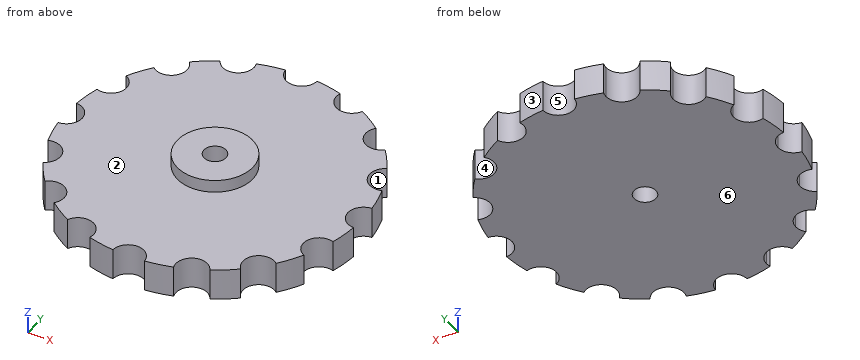
```python
from build123d import *

# Parameters (mm, degrees)
F1_DEPTH = 5
F2_R     = 6
F3_DEPTH = 2
F4_R     = 1.75
F5_DEPTH = 25


with BuildPart() as f1:
    # F0 (on Top) → F1 (new body)
    with BuildSketch(Plane.XY):
        with BuildLine():
            ThreePointArc((23.3670212736, -2.4964608548), (21, -2.53e-08), (23.3670212796, 2.4964607985))
            ThreePointArc((23.3670212796, 2.4964607985), (23.0484540943, 4.5846225431), (22.5436668971, 6.6357428244))
            ThreePointArc((22.5436668971, 6.6357428244), (19.40147019, 8.0363520621), (20.6329585055, 11.2486009491))
            ThreePointArc((20.6329585055, 11.2486009491), (19.5395358989, 13.0559004612), (18.2882435892, 14.7577148103))
            ThreePointArc((18.2882435892, 14.7577148103), (14.8492424139, 14.849242396), (14.7577148323, 18.2882435714))
            ThreePointArc((14.7577148323, 18.2882435714), (13.0559004848, 19.5395358832), (11.248600974, 20.6329584919))
            ThreePointArc((11.248600974, 20.6329584919), (8.0363520855, 19.4014701803), (6.6357428516, 22.5436668891))
            ThreePointArc((6.6357428516, 22.5436668891), (4.5846225709, 23.0484540888), (2.4964608267, 23.3670212766))
            ThreePointArc((2.4964608267, 23.3670212766), (0, 21), (-2.4964608267, 23.3670212766))
            ThreePointArc((-2.4964608267, 23.3670212766), (-4.5846225153, 23.0484540998), (-6.6357427429, 22.5436669211))
            ThreePointArc((-6.6357427429, 22.5436669211), (-6.5289892822, 22.1334873299), (-6.4930605625, 21.7111690547))
            ThreePointArc((-6.4930605625, 21.7111690547), (-8.440272529, 19.2730498225), (-11.2486008745, 20.6329585461))
            ThreePointArc((-11.2486008745, 20.6329585461), (-13.0559003906, 19.5395359461), (-14.7577147442, 18.2882436426))
            ThreePointArc((-14.7577147442, 18.2882436426), (-14.2826746546, 17.5119294358), (-14.1170092878, 16.617009428))
            ThreePointArc((-14.1170092878, 16.617009428), (-15.5991894549, 14.3335815688), (-18.2882435181, 14.7577148984))
            ThreePointArc((-18.2882435181, 14.7577148984), (-19.539535836, 13.0559005554), (-20.6329584512, 11.2486010486))
            ThreePointArc((-20.6329584512, 11.2486010486), (-19.5962781638, 10.3261912121), (-19.2111689788, 8.9930607456))
            ThreePointArc((-19.2111689788, 8.9930607456), (-20.267431592, 6.9520751117), (-22.5436668651, 6.6357429331))
            ThreePointArc((-22.5436668651, 6.6357429331), (-23.0484540722, 4.5846226542), (-23.3670212676, 2.4964609112))
            ThreePointArc((-23.3670212676, 2.4964609112), (-21.6858270712, 1.7201095537), (-21, 8.5e-08))
            ThreePointArc((-21, 8.5e-08), (-21.6858270774, -1.7201093903), (-23.3670212856, -2.4964607422))
            ThreePointArc((-23.3670212856, -2.4964607422), (-23.0484541054, -4.5846224875), (-22.5436669131, -6.6357427701))
            ThreePointArc((-22.5436669131, -6.6357427701), (-20.2674316496, -6.9520749599), (-19.2111690438, -8.9930605886))
            ThreePointArc((-19.2111690438, -8.9930605886), (-19.5962782336, -10.3261910627), (-20.6329585326, -11.2486008994))
            ThreePointArc((-20.6329585326, -11.2486008994), (-19.5395359304, -13.0559004141), (-18.2882436248, -14.7577147662))
            ThreePointArc((-18.2882436248, -14.7577147662), (-15.5991895668, -14.3335814524), (-14.1170094079, -16.6170093078))
            ThreePointArc((-14.1170094079, -16.6170093078), (-14.282674778, -17.5119293241), (-14.7577148764, -18.2882435359))
            ThreePointArc((-14.7577148764, -18.2882435359), (-13.0559005319, -19.5395358517), (-11.2486010237, -20.6329584648))
            ThreePointArc((-11.2486010237, -20.6329584648), (-8.4402726772, -19.2730497595), (-6.4930607194, -21.7111689896))
            ThreePointArc((-6.4930607194, -21.7111689896), (-6.5289894407, -22.1334872737), (-6.6357429059, -22.5436668731))
            ThreePointArc((-6.6357429059, -22.5436668731), (-4.5846226264, -23.0484540777), (-2.496460883, -23.3670212706))
            ThreePointArc((-2.496460883, -23.3670212706), (-5.06e-08, -21), (2.4964607704, -23.3670212826))
            ThreePointArc((2.4964607704, -23.3670212826), (4.5846225153, -23.0484540998), (6.6357427973, -22.5436669051))
            ThreePointArc((6.6357427973, -22.5436669051), (8.0363520388, -19.4014701997), (11.2486009242, -20.632958519))
            ThreePointArc((11.2486009242, -20.632958519), (13.0559004377, -19.5395359147), (14.7577147882, -18.288243607))
            ThreePointArc((14.7577147882, -18.288243607), (14.8492423781, -14.8492424318), (18.2882435536, -14.7577148544))
            ThreePointArc((18.2882435536, -14.7577148544), (19.5395358675, -13.0559005083), (20.6329584783, -11.2486009988))
            ThreePointArc((20.6329584783, -11.2486009988), (19.4014701706, -8.0363521089), (22.5436668811, -6.6357428788))
            ThreePointArc((22.5436668811, -6.6357428788), (23.0484540833, -4.5846225986), (23.3670212736, -2.4964608548))
        make_face()
    extrude(amount=F1_DEPTH)

    # F2 (on face) → F3 (join)
    with BuildSketch(Plane.XY.offset(5)):
        Circle(F2_R)
    extrude(amount=F3_DEPTH)

    # F4 (on face) → F5 (cut)
    with BuildSketch(Plane.XY.offset(7)):
        Circle(F4_R)
    extrude(amount=-F5_DEPTH, mode=Mode.SUBTRACT)


solid = f1.part
```
Design review of the part built by this model. Coordinates are the model's own, in mm. Face numbers are marked on the shaded views. A direction names the side the tool comes from. Round coordinates to 2 decimals unless told otherwise and drop trailing zeros. Order: outer loops, then holes, each group sorted by start corner. A loop starts at its lowest first (then second) coordinate and runs counter-clockwise, first axis right, second up. Notation, with made-up numbers: (22.25, 79) - (53.25, 79) arc R8 ccw to (53.25, 94) - close; hole circle Ø7 at (-21.75, 30.25). An arc over 180 degrees is marked (long way). One line per question, with ' | ' between items.
Item 1: Take a section at D-D, the plane x = 8. Write out the cut boundary in (y, z), then the cut area to 3 significant figures.
Checks:
outline: (-19.42, 0) - (19.42, 0) - (19.42, 5) - (-19.42, 5) - close | area: 194 mm²
Item 2: Machinability: for the marked faces 1 and 2, which of the approach directions +Z, -Z, +X, -X, +Y, -Y give a long, thin tool a straight path to every point of the face, cutting with its end or side? Answer none if there is none.
Checks:
face 1: +Z, -Z | face 2: +Z
Item 3: Draft analysis for pull direction X (two halves, no side actions). For the marked faces 3, 4, 5 and 6, state which applies: +X half, -X half, draft (parallel to the pull), parting line (faces both ways), or undercut.
Checks:
face 3: +X half | face 4: undercut | face 5: undercut | face 6: draft
Item 4: Take a section at A-A, the plane x = 0. Write out the cut boundary in (y, z), then the cut area to 4 significant figures.
Checks:
outline: (-21, 0) - (-1.75, 0) - (-1.75, 7) - (-6, 7) - (-6, 5) - (-21, 5) - close; (1.75, 0) - (21, 0) - (21, 5) - (6, 5) - (6, 7) - (1.75, 7) - close | area: 209.5 mm²
Item 5: Take a section at B-B, the plane x = 20. Write out the cut boundary in (y, z).
Checks:
outline: (-12.34, 0) - (-10.82, 0) - (-10.82, 5) - (-12.34, 5) - close; (-7.17, 0) - (7.17, 0) - (7.17, 5) - (-7.17, 5) - close; (10.82, 0) - (12.34, 0) - (12.34, 5) - (10.82, 5) - close
Item 6: Wall thickness on line 1 (Z direction, x = 0, y = -19); line 2 (Y direction, x = 17.5, z = 1.25); line 3 (X direction, y = 17, z = 2.75): over which ranges is each line inside the solid? List them lowest first. Write a range as [from, to].
Checks:
line 1: [0, 5] | line 2: [-14.28, 14.28] | line 3: [-14.15, 14.15]
Item 7: For P1, Ø2, axis at y = -7.5, z = 1.5, coming from the -X side; P2, Ø12, axis at x = 13.5, y = 11, coming from the +Z side, all flat-tipped, find the tip position at first contact; note any pin that passes through.
Checks:
P1: x = -22.58 | P2: z = 5
Item 8: Take a section at C-C, the plane x = -12. Write out the cut boundary in (y, z), then the cut area to 3 significant figures.
Checks:
outline: (-20.21, 0) - (20.21, 0) - (20.21, 5) - (-20.21, 5) - close | area: 202 mm²
